```python
from build123d import *

# Parameters (mm, degrees)
SKETCH1_W             = 24
SKETCH1_H             = 8
SKETCH1_R             = 1.075
BOSS_EXTRUDE1_DEPTH   = 5
BOSS_EXTRUDE1_2_DEPTH = 5
SKETCH2_W             = 50
SKETCH2_H             = 21
SKETCH2_R             = 1.075
BOSS_EXTRUDE2_DEPTH   = 8
BOSS_EXTRUDE3_DEPTH   = 10
CHAMFER1_SIZE         = 1
FILLET1_R             = 2
SKETCH3_R             = 1.15
CUT_EXTRUDE1_DEPTH    = 7


with BuildPart() as part:
    # Sketch1 → Boss-Extrude1 (new body)
    with BuildSketch(Plane.XY):
        with Locations((-8.500045519, -6.479626746)):
            Rectangle(SKETCH1_W, SKETCH1_H)
        with Locations((-14.500045519, -4.479626746)):
            Circle(SKETCH1_R, mode=Mode.SUBTRACT)
        with Locations((-2.500045519, -8.479626746)):
            Circle(SKETCH1_R, mode=Mode.SUBTRACT)
        with Locations(Location((-14.500045519, -8.479626746, 0), (0, 0, 180))):
            Circle(SKETCH1_R, mode=Mode.SUBTRACT)
        with Locations(Location((-2.500045519, -4.479626746, 0), (0, 0, 180))):
            Circle(SKETCH1_R, mode=Mode.SUBTRACT)
    extrude(amount=BOSS_EXTRUDE1_DEPTH)



with BuildPart() as body_2:
    # Sketch1 → Boss-Extrude1 2 (new body)
    with BuildSketch(Plane.XY):
        with Locations((17.499954481, 6.520373254)):
            Rectangle(SKETCH1_W, SKETCH1_H)
        with Locations((11.499954481, 8.520373254)):
            Circle(SKETCH1_R, mode=Mode.SUBTRACT)
        with Locations(Location((11.499954481, 4.520373254, 0), (0, 0, 180))):
            Circle(SKETCH1_R, mode=Mode.SUBTRACT)
        with Locations((23.499954481, 4.520373254)):
            Circle(SKETCH1_R, mode=Mode.SUBTRACT)
        with Locations(Location((23.499954481, 8.520373254, 0), (0, 0, 180))):
            Circle(SKETCH1_R, mode=Mode.SUBTRACT)
    extrude(amount=BOSS_EXTRUDE1_2_DEPTH)


with BuildPart() as part_1:
    add(part.part)

    add(body_2.part)  # Boss-Extrude2 merges body 2
    # Sketch2 → Boss-Extrude2 (add)
    with BuildSketch(Plane.XY.offset(5)):
        with Locations((4.499954481, 0.020373254)):
            Rectangle(SKETCH2_W, SKETCH2_H)
        with Locations((-14.500045519, -8.479626746)):
            Circle(SKETCH2_R, mode=Mode.SUBTRACT)
        with Locations((-2.500045519, -8.479626746)):
            Circle(SKETCH2_R, mode=Mode.SUBTRACT)
        with Locations((-14.500045519, -4.479626746)):
            Circle(SKETCH2_R, mode=Mode.SUBTRACT)
        with Locations((-2.500045519, -4.479626746)):
            Circle(SKETCH2_R, mode=Mode.SUBTRACT)
        with Locations((23.499954481, 8.520373254)):
            Circle(SKETCH2_R, mode=Mode.SUBTRACT)
        with Locations((11.499954481, 8.520373254)):
            Circle(SKETCH2_R, mode=Mode.SUBTRACT)
        with Locations((11.499954481, 4.520373254)):
            Circle(SKETCH2_R, mode=Mode.SUBTRACT)
        with Locations((23.499954481, 4.520373254)):
            Circle(SKETCH2_R, mode=Mode.SUBTRACT)
    extrude(amount=BOSS_EXTRUDE2_DEPTH)

    # Sketch2<6> → Boss-Extrude3 (add)
    with BuildSketch(Plane.XY.offset(5)):
        Polygon((3.499954481, -2.479626746), (3.499954481, -10.479626746), (29.499954481, -10.479626746), (29.499954481, 2.520373254), (5.499954481, 2.520373254), (5.499954481, 10.520373254), (-20.500045519, 10.520373254), (-20.500045519, -2.479626746), align=None)
    extrude(amount=BOSS_EXTRUDE3_DEPTH)

    # Chamfer1
    # the kernel refuses this chamfer: 1 mm, written as the material it takes off along each edge
    with BuildSketch(Plane(origin=(23.499954481, 8.520373254, 13), x_dir=(1, 0, 0), z_dir=(0, -1, 0))) as chamfer1_piece_1:
        Polygon((1.075 + CHAMFER1_SIZE, 0), (1.075, -CHAMFER1_SIZE), (1.075, 0), align=None)
    revolve(axis=Axis((23.499954481, 8.520373254, 13), (0, 0, 1)), mode=Mode.SUBTRACT)
    with BuildSketch(Plane(origin=(11.499954481, 4.520373254, 13), x_dir=(1, 0, 0), z_dir=(0, -1, 0))) as chamfer1_piece_2_section:
        Polygon((1.075 + CHAMFER1_SIZE, 0), (1.075, -CHAMFER1_SIZE), (1.075, 0), align=None)
    chamfer1_piece_2 = revolve(axis=Axis((11.499954481, 4.520373254, 13), (0, 0, 1)), mode=Mode.PRIVATE)
    chamfer1_piece_2 = split(chamfer1_piece_2, bisect_by=Plane(origin=(9.93692483, 2.520373254, 12.511970349), z_dir=(0, 1, 0)), keep=Keep.TOP, mode=Mode.PRIVATE)
    add(chamfer1_piece_2, mode=Mode.SUBTRACT)
    with BuildSketch(Plane(origin=(11.499954481, 8.520373254, 13), x_dir=(1, 0, 0), z_dir=(0, -1, 0))) as chamfer1_piece_3:
        Polygon((1.075 + CHAMFER1_SIZE, 0), (1.075, -CHAMFER1_SIZE), (1.075, 0), align=None)
    revolve(axis=Axis((11.499954481, 8.520373254, 13), (0, 0, 1)), mode=Mode.SUBTRACT)
    with BuildSketch(Plane(origin=(23.499954481, 4.520373254, 13), x_dir=(1, 0, 0), z_dir=(0, -1, 0))) as chamfer1_piece_4_section:
        Polygon((1.075 + CHAMFER1_SIZE, 0), (1.075, -CHAMFER1_SIZE), (1.075, 0), align=None)
    chamfer1_piece_4 = revolve(axis=Axis((23.499954481, 4.520373254, 13), (0, 0, 1)), mode=Mode.PRIVATE)
    chamfer1_piece_4 = split(chamfer1_piece_4, bisect_by=Plane(origin=(21.93692483, 2.520373254, 12.511970349), z_dir=(0, 1, 0)), keep=Keep.TOP, mode=Mode.PRIVATE)
    add(chamfer1_piece_4, mode=Mode.SUBTRACT)
    with BuildSketch(Plane(origin=(-14.500045519, -4.479626746, 13), x_dir=(1, 0, 0), z_dir=(0, -1, 0))) as chamfer1_piece_5_section:
        Polygon((1.075 + CHAMFER1_SIZE, 0), (1.075, -CHAMFER1_SIZE), (1.075, 0), align=None)
    chamfer1_piece_5 = revolve(axis=Axis((-14.500045519, -4.479626746, 13), (0, 0, 1)), mode=Mode.PRIVATE)
    chamfer1_piece_5 = split(chamfer1_piece_5, bisect_by=Plane(origin=(-16.063075173, -2.479626746, 12.511970346), z_dir=(0, -1, 0)), keep=Keep.TOP, mode=Mode.PRIVATE)
    add(chamfer1_piece_5, mode=Mode.SUBTRACT)
    with BuildSketch(Plane(origin=(-14.500045519, -8.479626746, 13), x_dir=(1, 0, 0), z_dir=(0, -1, 0))) as chamfer1_piece_6:
        Polygon((1.075 + CHAMFER1_SIZE, 0), (1.075, -CHAMFER1_SIZE), (1.075, 0), align=None)
    revolve(axis=Axis((-14.500045519, -8.479626746, 13), (0, 0, 1)), mode=Mode.SUBTRACT)
    with BuildSketch(Plane(origin=(-2.500045519, -4.479626746, 13), x_dir=(1, 0, 0), z_dir=(0, -1, 0))) as chamfer1_piece_7_section:
        Polygon((1.075 + CHAMFER1_SIZE, 0), (1.075, -CHAMFER1_SIZE), (1.075, 0), align=None)
    chamfer1_piece_7 = revolve(axis=Axis((-2.500045519, -4.479626746, 13), (0, 0, 1)), mode=Mode.PRIVATE)
    chamfer1_piece_7 = split(chamfer1_piece_7, bisect_by=Plane(origin=(-4.063075173, -2.479626746, 12.511970346), z_dir=(0, -1, 0)), keep=Keep.TOP, mode=Mode.PRIVATE)
    add(chamfer1_piece_7, mode=Mode.SUBTRACT)
    with BuildSketch(Plane(origin=(-2.500045519, -8.479626746, 13), x_dir=(1, 0, 0), z_dir=(0, -1, 0))) as chamfer1_piece_8:
        Polygon((1.075 + CHAMFER1_SIZE, 0), (1.075, -CHAMFER1_SIZE), (1.075, 0), align=None)
    revolve(axis=Axis((-2.500045519, -8.479626746, 13), (0, 0, 1)), mode=Mode.SUBTRACT)

    # Fillet1
    fillet1_edges = [part_1.edges().sort_by_distance(p)[0] for p in [
        (29.499954481, -10.479626746, 9),
        (29.499954481, 10.520373254, 9),
        (-20.500045519, 10.520373254, 10),
        (-20.500045519, -10.479626746, 6.5),
    ]]
    fillet(fillet1_edges, radius=FILLET1_R)

    # Sketch3 → Cut-Extrude1 (cut)
    with BuildSketch(Plane.XY.offset(15)):
        with Locations((4.499954481, 0.020373254)):
            Circle(SKETCH3_R)
        with Locations((24.499954481, 0.020373254)):
            Circle(SKETCH3_R)
        with Locations((-15.500045519, 0.020373254)):
            Circle(SKETCH3_R)
        with Locations((-15.500045519, 7.020373254)):
            Circle(SKETCH3_R)
        with Locations((-5.500045519, 7.020373254)):
            Circle(SKETCH3_R)
        with Locations((14.499954481, -6.979626746)):
            Circle(SKETCH3_R)
        with Locations((24.499954481, -6.979626746)):
            Circle(SKETCH3_R)
    extrude(amount=-CUT_EXTRUDE1_DEPTH, mode=Mode.SUBTRACT)


solid = part_1.part
```
For this review, take the finished solid that the model builds, in its own axes (mm). A direction names the side the tool comes from. Give positions to 0.01 mm unless a question says otherwise; leave off trailing zeros. Write each loop counter-clockwise with the first axis right and the second up, starting at its lowest first coordinate (ties: lowest second). Pieces come first, ordered by that corner, then holes. Notation, with made-up numbers: M 67.5,88.5 L 80.5,88.5 A19 cw 80.5,123.5 Z; hole C 28,-11 d5. An arc over 180 degrees is marked long. Answer as a JSON object with one key per item and string values. Group by question number.
Item 1: For probe 1 along Y at (x, z) = (11.5, 8); probe 2 along X at (y, z) = (-7.5, 5.5); probe 3 along X at (y, z) = (8.25, 0.5), list the stretches that pass through material, from the lowest coordinate up. Write a range as [from, to].
Item 2: Consider section A-A on z = 3.75. Count the separate pieces of the cut face and the enclosed holes in it, plus the area to 3 significant figures.
Item 3: Tool access review of faces 5 (the flat face through (4, 0, 5)), 6 (the flat face through (3.5, -6, 14)), 7 (the flat face through (4, 3, 15)), 8 (the flat face through (-16, 0, 8)): name each direction out of +Z, -Z, +X, -X, +Y, -Y from which nothing blocks a thin tool from reaching the whole face with its end or side.
Item 4: Consider section B-B on x = 8. Write out the cut boundary in (y, z), plus the area to 3 significant figures.
Item 5: For pin 1 Ø2.5 at (x, y) = (-14.5, -4.48) entering from +Z; pin 2 Ø3 at (x, y) = (24.5, 0.02) entering from -Z; pin 3 Ø1.8 at (x, y) = (-5.5, 7.02) entering from +Z, all flat-tipped, find the tip position at first contact; note any pin that passes through.
Item 6: Draft analysis for pull direction X (two halves, no side actions). For faces 1 (the cylindrical face through (-19.93, 9.92, 9.93)), 2 (the flat face through (17, 7, 0)), 3 (the cylindrical face through (-16.348, 7.798, 11.549)), 4 (the cylindrical face through (28.9, -9.91, 10.07)), state which applies: +X half, -X half, draft (parallel to the pull), parting line (faces both ways), or undercut.
Item 7: Consider section C-C on y = -0.5. Write out the cut boundary in (x, z).
Check result:
{
 "1": {"probe 1": "y = [-10.48, 3.45], [5.6, 7.45], [9.6, 10.52]", "probe 2": "x = [-20.5, -14.94], [-14.06, -2.94], [-2.06, 29.5]", "probe 3": "x = [5.5, 10.46], [12.54, 22.46], [24.54, 29.5]"},
 "2": {"separate pieces": "2", "enclosed holes": "8", "area": "353 mm^2"},
 "3": {"face 5": "-Z", "face 6": "+Z, -X, -Y", "face 7": "+Z, +X, -X, +Y, -Y", "face 8": "+Z"},
 "4": {"outline": "M -10.48,5 L 2.52,5 L 2.52,0 L 10.52,0 L 10.52,13 L 2.52,13 L 2.52,15 L -10.48,15 Z", "area": "234 mm^2"},
 "5": {"pin 1": "stops at z = 12.18", "pin 2": "stops at z = 5", "pin 3": "stops at z = 8"},
 "6": {"face 1": "-X half", "face 2": "draft", "face 3": "undercut", "face 4": "+X half"},
 "7": {"outline": "M -20.5,5 L 29.5,5 L 29.5,15 L 25.53,15 L 25.53,8 L 23.47,8 L 23.47,15 L 5.53,15 L 5.53,8 L 3.47,8 L 3.47,15 L -14.47,15 L -14.47,8 L -16.53,8 L -16.53,15 L -20.5,15 Z"}
}
